For this review, take the finished solid that the model builds, in its own axes (mm). Round coordinates to 2 decimals unless told otherwise and drop trailing zeros. Write each loop counter-clockwise with the first axis right and the second up, starting at its lowest first coordinate (ties: lowest second). Pieces come first, ordered by that corner, then holes. Notation, with made-up numbers: (9, 60.5) - (67, 60.5) arc R28 ccw to (67, 93.5) - close; hole circle Ø8 at (5.5, 13.25). An arc over 180 degrees is marked (long way). One line per item, written item: value. Start each with the question number.
Q1. Add section B-B on x = -30.75. Write out the cut boundary in (y, z).
Q2. Mouldability with a two-part tool opening along X and no side actions: class faces 1 (the face through (-20.69, 2.54, 34.16)), 2 (the face through (-31.94, 2.54, 8.41)), 3 (the face through (-33.75, 3, -1)), 4 (the face through (0, 2, 42.5)) as +X half, -X half, draft (parallel to the pull), parting line (faces both ways), or undercut.
Q3. Clearance check with a flat-ended pin moving along its axis: pin 1 Ø3.5 at (x, z) = (-30.75, 7.5) entering from -Y. State where the tip first meets the part, or that it passes through.
Q4. Add section A-A on z = 19.75. Write out the cut boundary in (x, y).
Q5. For probe 1 along X at (y, z) = (3.25, 7.5); probe 2 along X at (y, z) = (3.5, 33.25); probe 3 along X at (y, z) = (3.15, 34), list the stretches that pass through material, from the lowest coordinate up.
```python
from build123d import *

# Parameters (mm, degrees)
SKETCH1_W           = 66
SKETCH1_H           = 85
BOSS_EXTRUDE1_DEPTH = 5
SKETCH4_R           = 1.5
CUT_EXTRUDE2_DEPTH  = 10
SKETCH8_W           = 85
SKETCH8_H           = 5
BOSS_EXTRUDE2_DEPTH = 0.75
SKETCH9_W           = 85
SKETCH9_H           = 5
BOSS_EXTRUDE3_DEPTH = 0.75
SKETCH10_R          = 1.5
CUT_EXTRUDE3_DEPTH  = 10


with BuildPart() as part:
    # Sketch1 → Boss-Extrude1 (new body)
    with BuildSketch(Plane(origin=(0, 0, 0), x_dir=(1, 0, 0), z_dir=(0, 1, 0))):
        Rectangle(SKETCH1_W, SKETCH1_H)
    extrude(amount=BOSS_EXTRUDE1_DEPTH)

    # Sketch4 → Cut-Extrude2 (cut)
    with BuildSketch(Plane(origin=(0, 5, 0), x_dir=(1, 0, 0), z_dir=(0, 1, 0))):
        with Locations((-30.75, 7.5)):
            Circle(SKETCH4_R)
        with Locations((-14.75, 7.5)):
            Circle(SKETCH4_R)
        with Locations((-30.75, -7.5)):
            Circle(SKETCH4_R)
        with Locations((-14.75, -7.5)):
            Circle(SKETCH4_R)
        with Locations((14.75, -7.5)):
            Circle(SKETCH4_R)
        with Locations((30.75, -7.5)):
            Circle(SKETCH4_R)
        with Locations((14.75, 7.5)):
            Circle(SKETCH4_R)
        with Locations((30.75, 7.5)):
            Circle(SKETCH4_R)
    extrude(amount=-CUT_EXTRUDE2_DEPTH, mode=Mode.SUBTRACT)

    # Sketch8 → Boss-Extrude2 (add)
    with BuildSketch(Plane.ZY.offset(33)):
        with Locations((0, 2.5)):
            Rectangle(SKETCH8_W, SKETCH8_H)
    extrude(amount=BOSS_EXTRUDE2_DEPTH)

    # Sketch9 → Boss-Extrude3 (add)
    with BuildSketch(Plane(origin=(33, 0, 0), x_dir=(0, 0, -1), z_dir=(1, 0, 0))):
        with Locations((0, 2.5)):
            Rectangle(SKETCH9_W, SKETCH9_H)
    extrude(amount=BOSS_EXTRUDE3_DEPTH)

    # Sketch10 → Cut-Extrude3 (cut)
    with BuildSketch(Plane(origin=(0, 5, 0), x_dir=(1, 0, 0), z_dir=(0, 1, 0))):
        with Locations((-19.5, -33.25)):
            Circle(SKETCH10_R)
        with Locations((-19.5, -19.75)):
            Circle(SKETCH10_R)
        with Locations((19.5, -33.25)):
            Circle(SKETCH10_R)
        with Locations((19.5, -19.75)):
            Circle(SKETCH10_R)
    extrude(amount=-CUT_EXTRUDE3_DEPTH, mode=Mode.SUBTRACT)


solid = part.part
```
Result set:
1. outline: (0, -42.5) - (5, -42.5) - (5, -9) - (0, -9) - close; (0, -6) - (5, -6) - (5, 6) - (0, 6) - close; (0, 9) - (5, 9) - (5, 42.5) - (0, 42.5) - close
2. face 1: undercut
2. face 2: undercut
2. face 3: -X half
2. face 4: draft
3. pin 1: stops at y = 0
4. outline: (-33.75, 0) - (-21, 0) - (-21, 5) - (-33.75, 5) - close; (-18, 0) - (18, 0) - (18, 5) - (-18, 5) - close; (21, 0) - (33.75, 0) - (33.75, 5) - (21, 5) - close
5. probe 1: x = -33.75 to -32.25, -29.25 to -16.25, -13.25 to 13.25, 16.25 to 29.25, 32.25 to 33.75
5. probe 2: x = -33.75 to -21, -18 to 18, 21 to 33.75
5. probe 3: x = -33.75 to -20.8, -18.2 to 18.2, 20.8 to 33.75
